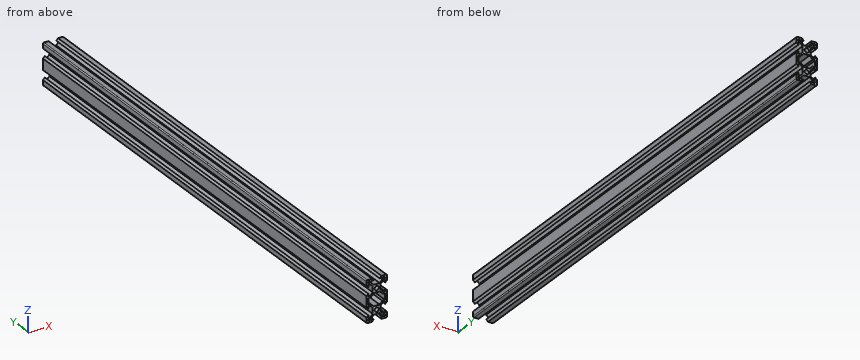
from build123d import *

# Parameters (mm, degrees)
F0_W             = 20
F0_H             = 20
F1_DEPTH         = 488
F2_R             = 2.1
F3_DEPTH         = 488.001
F4_R             = 1
F6_DEPTH         = 488.001
F6_COPIES3_COUNT = 2
F6_COPIES3_ANGLE = 90
F6_COPIES4_COUNT = 2
F6_COPIES4_ANGLE = 270
F6_COPIES6_COUNT = 2
F9_W             = 16.4
F9_H             = 6.8613203436
F10_DEPTH        = 488.001
F12_DEPTH        = 488


# Not quite as in the source:
# - a pattern or mirror of a feature is missing from the dataset's text; its kind, count and spacing are read off the source's solid


with BuildPart() as f1:
    # F0 (on Front) → F1 (new body)
    with BuildSketch(Plane.XZ):
        Rectangle(F0_W, F0_H)
    extrude(amount=F1_DEPTH)

    # F2 (on face) → F3 (cut, through all)
    with BuildSketch(Plane.XZ.offset(488)):
        Circle(F2_R)
    extrude(amount=-F3_DEPTH, mode=Mode.SUBTRACT)

    # F4
    f4_edges = [f1.edges().sort_by_distance(p)[0] for p in [
        (-10, -244, 10),
        (10, -244, 10),
    ]]
    fillet(f4_edges, radius=F4_R)

    # F5 (on face) → F6 (cut, through all)
    with BuildSketch(Plane.XZ.offset(488)):
        Polygon((0, 3.9006601718), (0, 10), (-2.84, 10), (-4.64, 10), (-2.84, 8.2), (-5.4993398282, 8.2), (-5.4993398282, 6.56), (-2.84, 3.9006601718), align=None)
        Polygon((-6.5693398282, 8.2), (-8.2, 8.2), (-7.0953059148, 7.0953059148), (-6.5693398282, 7.6212720014), align=None)
    f6 = extrude(amount=-F6_DEPTH, mode=Mode.SUBTRACT)

    # F6_copies: F6 across plane
    add(f6.mirror(Plane(origin=(0, 0, 0), x_dir=(-0.7071067812, 0, -0.7071067812), z_dir=(0.7071067812, 0, -0.7071067812))), mode=Mode.SUBTRACT)

    # F6_copies1: F6 across plane
    add(f6.mirror(Plane(origin=(0, 0, 0), x_dir=(0.7071067812, 0, -0.7071067812), z_dir=(-0.7071067812, 0, -0.7071067812))), mode=Mode.SUBTRACT)

    # F6_copies2: F6 across plane
    add(f6.mirror(Plane(origin=(0, 0, 0), x_dir=(0, 0, 1), z_dir=(1, 0, 0))), mode=Mode.SUBTRACT)

    # F6_copies3: F6 ×2 about axis
    f6_copies3_axis = Axis((0, 0, 0), (0, 1, 0))
    for i in range(1, F6_COPIES3_COUNT):
        add(f6.rotate(f6_copies3_axis, i * F6_COPIES3_ANGLE / (F6_COPIES3_COUNT - 1)), mode=Mode.SUBTRACT)

    # F6_copies4: F6 ×2 about axis
    f6_copies4_axis = Axis((0, 0, 0), (0, 1, 0))
    for i in range(1, F6_COPIES4_COUNT):
        add(f6.rotate(f6_copies4_axis, i * F6_COPIES4_ANGLE / (F6_COPIES4_COUNT - 1)), mode=Mode.SUBTRACT)

    # F6_copies5: F6 across plane
    add(f6.mirror(Plane(origin=(0, 0, 0), x_dir=(-1, 0, 0), z_dir=(0, 0, -1))), mode=Mode.SUBTRACT)

    # F6_copies6: F6 ×2 about axis
    f6_copies6_axis = Axis((0, 0, 0), (0, 1, 0))
    for i in range(1, F6_COPIES6_COUNT):
        add(f6.rotate(f6_copies6_axis, i * 360 / F6_COPIES6_COUNT), mode=Mode.SUBTRACT)

    # F8: F1 across face


with BuildPart() as f1_1:
    add(f1.part)
    add(f1.part.mirror(Plane(origin=(-7.32, -244, -10), x_dir=(1, 0, 0), z_dir=(0, 0, -1))))

    # F9 (on face) → F10 (cut, through all)
    with BuildSketch(Plane.XZ.offset(488)):
        with Locations((0, -10)):
            Rectangle(F9_W, F9_H)
    extrude(amount=-F10_DEPTH, mode=Mode.SUBTRACT)

    # F11 (on face) → F12 (join, through all)
    with BuildSketch(Plane.XZ.offset(488)):
        with BuildLine():
            ThreePointArc((-9, -10), (-9.7071067812, -9.7071067812), (-10, -9))
            Line((-10, -9), (-10, -11))
            ThreePointArc((-10, -11), (-9.7071067812, -10.2928932188), (-9, -10))
        make_face()
        with BuildLine():
            ThreePointArc((10, -9), (9.7071067812, -9.7071067812), (9, -10))
            ThreePointArc((9, -10), (9.7071067812, -10.2928932188), (10, -11))
            Line((10, -11), (10, -9))
        make_face()
        Polygon((5.9386796564, -6.9993398282), (8.2, -6.9993398282), (8.2, -6.5693398282), (5.5086796564, -6.5693398282), align=None)
        Polygon((-8.2, -6.5693398282), (-8.2, -6.9993398282), (-5.9386796564, -6.9993398282), (-5.5086796564, -6.5693398282), align=None)
    extrude(amount=-F12_DEPTH)


solid = f1_1.part
Read the model definition and answer for the solid it produces. Units are mm, in the model's axes. Round coordinates to 2 decimals unless told otherwise and drop trailing zeros.
Q1. Consider probe 1 along Z at (x, y) = (0, -325); probe 2 along Z at (x, y) = (9.25, -332.5); probe 3 along X at (y, z) = (-429.5, -9.5). Determine where each line is inside the solid, lowest interval first.
Q2. Each of these flat-tipped pins is pushed along its axis until it touches: pin 1 (0.8 mm diameter, centred on y = -287, z = -4, fed in from -X); pin 2 (4.5 mm diameter, centred on x = -0.5, y = -336.5, fed in from -Z); pin 3 (0.8 mm diameter, centred on y = -224, z = -23.5, fed in from +X). Where does it stop, or does it pass through?
Q3. Section A-A on y = -141 is taken. Give the number of separate pieces and of enclosed holes in the cut face, and give its area (3 significant figures).
Output:
1. probe 1: z = -23.9 to -22.1, -17.9 to -16.1, -3.9 to -2.1, 2.1 to 3.9
1. probe 2: z = -29.97 to -23.89, -16.11 to -3.89, 3.89 to 9.97
1. probe 3: x = -10 to -8.2, 8.2 to 10
2. pin 1: stops at x = -9.76
2. pin 2: stops at z = -23.9
2. pin 3: stops at x = 9.26
3. separate pieces: 1
3. enclosed holes: 7
3. area: 286 mm2
